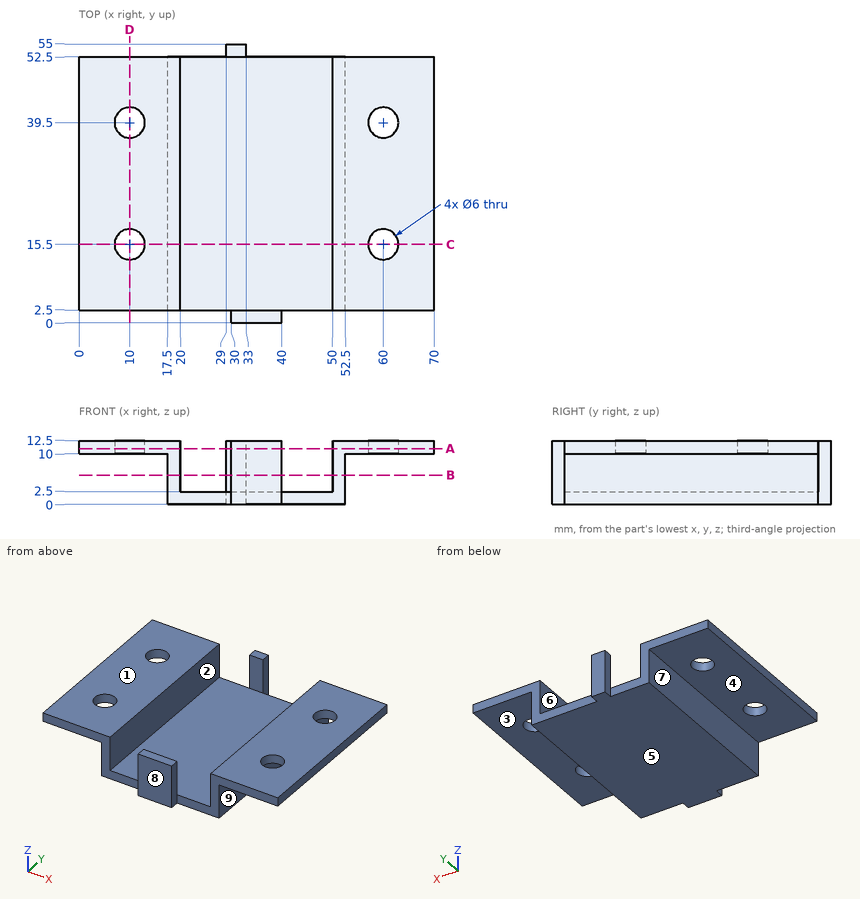
Drawing for the job (mm, zero at the part's lowest x, y, z). A direction names the side the tool comes from. Give positions to 0.01 mm unless a question says otherwise; leave off trailing zeros. Order: outer loops, then holes, each group sorted by start corner. A loop starts at its lowest first (then second) coordinate and runs counter-clockwise, first axis right, second up. Notation, with made-up numbers: M 58.25,-2 L 71.25,-2 A16 cw 71.25,22 Z; hole C -24.75,-6.75 d10. An arc over 180 degrees is marked long. Put each result on its own line as item: value.
Item 1: Slice it at D-D, the plane x = 10. Write the cut outline in (y, z).
From the geometry:
outline: M 2.5,10 L 12.5,10 L 12.5,12.5 L 2.5,12.5 Z; M 18.5,10 L 36.5,10 L 36.5,12.5 L 18.5,12.5 Z; M 42.5,10 L 52.5,10 L 52.5,12.5 L 42.5,12.5 Z
Item 2: Flat gauge pins, fed straight in: pin 1 Ø5.5 at (x, y) = (60, 15.5) entering from +Z; pin 2 Ø3 at (y, z) = (8.5, 7.5) entering from +X; pin 3 Ø3 at (y, z) = (53.5, 8.5) entering from -X; pin 4 Ø4 at (x, z) = (60, 11) entering from -Y. Where does each tip first touch, or does it go through?
From the geometry:
pin 1: passes through
pin 2: stops at x = 52.5
pin 3: stops at x = 17.5
pin 4: stops at y = 2.5
Item 3: Slice it at A-A, the plane z = 11. Write the cut outline in (x, y).
From the geometry:
outline: M 0,2.5 L 20,2.5 L 20,52.5 L 0,52.5 Z; M 29,52.5 L 33,52.5 L 33,55 L 29,55 Z; M 30,0 L 40,0 L 40,2.5 L 30,2.5 Z; M 50,2.5 L 70,2.5 L 70,52.5 L 50,52.5 Z; hole C 10,15.5 d6; hole C 10,39.5 d6; hole C 60,15.5 d6; hole C 60,39.5 d6
Item 4: Probe line 1 (Y direction, x = 60, z = 11.3); line 2 (X direction, y = 50, z = 10.5); line 3 (X direction, y = 13, z = 5.25). List the from-to ranges inside material, lowest first. Write a range as [from, to].
From the geometry:
line 1: y = [2.5, 12.5], [18.5, 36.5], [42.5, 52.5]
line 2: x = [0, 20], [50, 70]
line 3: x = [17.5, 20], [50, 52.5]
Item 5: Slice it at B-B, the plane z = 5.75. Write the cut outline in (x, y), plus the area to 3 significant figures.
From the geometry:
outline: M 17.5,2.5 L 20,2.5 L 20,52.5 L 17.5,52.5 Z; M 29,52.5 L 33,52.5 L 33,55 L 29,55 Z; M 30,0 L 40,0 L 40,2.5 L 30,2.5 Z; M 50,2.5 L 52.5,2.5 L 52.5,52.5 L 50,52.5 Z
area: 285 mm2
Item 6: 3-axis set-ups, long thin cutter, end or side, ignore diameter. For the marked faces 1, 2, 3, 4 and 5: which of +Z, -Z, +X, -X, +Y, -Y reach the whole face in a straight line?
From the geometry:
face 1: +Z, +X, -X, +Y, -Y
face 2: +Z, +Y, -Y
face 3: -Z, +X, +Y, -Y
face 4: -Z, -X, +Y, -Y
face 5: -Z, +X, -X, +Y, -Y
Item 7: Two-plate mould, pull along X, no slides. Class the marked faces 6, 7, 8 and 9: +X half, -X half, draft (parallel to the pull), parting line (faces both ways), or undercut.
From the geometry:
face 6: undercut
face 7: -X half
face 8: draft
face 9: +X half
Item 8: Slice it at C-C, the plane y = 15.5. Write the cut outline in (x, z).
From the geometry:
outline: M 0,10 L 7,10 L 7,12.5 L 0,12.5 Z; M 13,10 L 17.5,10 L 17.5,0 L 52.5,0 L 52.5,10 L 57,10 L 57,12.5 L 50,12.5 L 50,2.5 L 20,2.5 L 20,12.5 L 13,12.5 Z; M 63,10 L 70,10 L 70,12.5 L 63,12.5 Z
